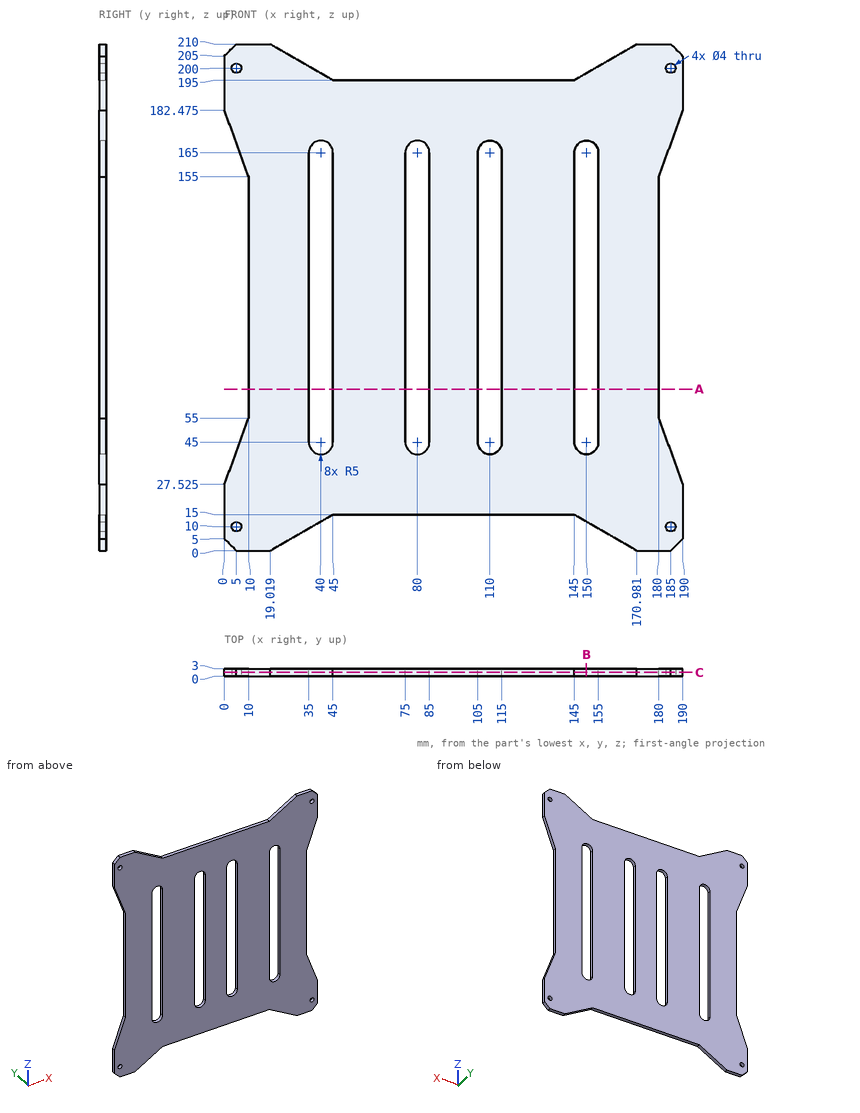
Geometry: see drawing. Coordinates: mm, zero at the bounding-box minimum. Give positions to 0.01 mm unless a question says otherwise; leave off trailing zeros. Write each loop counter-clockwise with the first axis right and the second up, starting at its lowest first coordinate (ties: lowest second). Pieces come first, ordered by that corner, then holes. Notation, with made-up numbers: (-29, 56) - (-16, 56) arc R20 ccw to (-16, 82) - close; hole circle Ø1 at (32.25, 75.5). An arc over 180 degrees is marked (long way). Return JSON: item names as keys, results as strings. Group by question number.
1) Section B-B on x = 150. Return the cut outline in (y, z).
2) Line query: line 1 (X direction, y = 1.6, z = 146); line 2 (X direction, y = 2.15, z = 10); line 3 (X direction, y = 2.05, z = 167). Output: solid intervals per line, ascending.
3) First-contact query: P1, Ø0.9, axis at y = 2, z = 124.5, coming from the -X side; P2, Ø1.5, axis at y = 1.5, z = 109.5, coming from the +X side; P3, Ø1, axis at x = 75, y = 2.5, coming from the +Z side. Flat tips, straight axial feed; report the tip coordinate or a pass-through.
4) Section A-A on z = 67. Return the cut outline in (x, y).
5) Section C-C on y = 1.5. State how many separate pieces and enclosed holes the cut face has, plus the area to 3 significant figures.
Filled in:
{
 "1": {"outline": "(0, 12.11) - (3, 12.11) - (3, 40) - (0, 40) - close; (0, 170) - (3, 170) - (3, 197.89) - (0, 197.89) - close"},
 "2": {"line 1": "x = 10 to 35, 45 to 75, 85 to 105, 115 to 145, 155 to 180", "line 2": "x = 0 to 3, 7 to 36.34, 153.66 to 183, 187 to 190", "line 3": "x = 5.63 to 35.42, 44.58 to 75.42, 84.58 to 105.42, 114.58 to 145.42, 154.58 to 184.37"},
 "3": {"P1": "stops at x = 10", "P2": "stops at x = 180", "P3": "stops at z = 195"},
 "4": {"outline": "(10, 0) - (35, 0) - (35, 3) - (10, 3) - close; (45, 0) - (75, 0) - (75, 3) - (45, 3) - close; (85, 0) - (105, 0) - (105, 3) - (85, 3) - close; (115, 0) - (145, 0) - (145, 3) - (115, 3) - close; (155, 0) - (180, 0) - (180, 3) - (155, 3) - close"},
 "5": {"separate pieces": "1", "enclosed holes": "8", "area": "28,400 mm^2"}
}
